Check sheet for the modelled part. Datum: model origin and axes. Units: mm. A direction names the side the tool comes from. Coordinates: 2 decimals unless noted, no trailing zeros. Order: outer loops, then holes, each group sorted by start corner. A loop starts at its lowest first (then second) coordinate and runs counter-clockwise, first axis right, second up. Notation, with made-up numbers: (83, 16.5) -> (114, 16.5) arc R25 cw to (114, 42.5) -> close; hole circle Ø6 at (87, 44). An arc over 180 degrees is marked (long way). Put each result on its own line as item: value. Start each with the question number.
```python
from build123d import *

# Parameters (mm, degrees)
F0_W     = 254
F0_H     = 254
F0_R     = 12.7
F1_DEPTH = 38.1
F2_W     = 254
F2_H     = 254
F2_W_2   = 241.3
F2_H_2   = 241.3
F3_DEPTH = 25.4
F4_R     = 19.05
F5_DEPTH = 37.846
F7_DEPTH = 50.8
F9_DEPTH = 50.8


with BuildPart() as f1:
    # F0 (on Top) → F1 (new body)
    with BuildSketch(Plane.XY):
        Rectangle(F0_W, F0_H)
        Circle(F0_R, mode=Mode.SUBTRACT)
    extrude(amount=-F1_DEPTH)

    # F2 (on face) → F3 (join)
    with BuildSketch(Plane.XY):
        Rectangle(F2_W, F2_H)
        Rectangle(F2_W_2, F2_H_2, mode=Mode.SUBTRACT)
    extrude(amount=F3_DEPTH)

    # F4 (on face) → F5 (cut)
    with BuildSketch(Plane.XY):
        Circle(F4_R)
    extrude(amount=-F5_DEPTH, mode=Mode.SUBTRACT)

    # F6 (on face) → F7 (join)
    with BuildSketch(Plane.YZ.offset(127)):
        Polygon((203.2, -170.082272), (127, -38.1), (76.2, -38.1), (152.4, -170.082272), align=None)
        Polygon((-76.2, -38.1), (-127, -38.1), (-203.2, -170.082272), (-152.4, -170.082272), align=None)
    extrude(amount=-F7_DEPTH)

    # F8 (on face) → F9 (join)
    with BuildSketch(Plane(origin=(-127, 0, 0), x_dir=(0, -1, 0), z_dir=(-1, 0, 0))):
        Polygon((-76.2, -38.1), (-127, -38.1), (-203.2, -170.082272), (-152.4, -170.082272), align=None)
        Polygon((203.2, -170.082272), (127, -38.1), (76.2, -38.1), (152.4, -170.082272), align=None)
    extrude(amount=-F9_DEPTH)


solid = f1.part
```
1) Access from +Z, -Z, +X, -X, +Y, -Y to the whole of each face (thin tool, end or side, straight path). Record for faces 1 (the flat face through (26, 2, -38.1)), 2 (the flat face through (76.2, -141, -103)), 3 (the flat face through (-29, 2, 0)), 4 (the flat face through (-101.956, 114.833, -105.015)), 5 (the flat face through (-2, -127, -7)).
2) Sectioned sample at D-D (x = -72). Record the boundary of the cut face in (y, z), plus the area to 4 significant figures.
3) Mould release check, pull along X, two halves, no side actions. Record for faces 6 (the flat face through (101.96, 113.77, -103.17)), 7 (the flat face through (-127, 1, -21)), 8 (the flat face through (-76.2, 141, -103)): +X half, -X half, draft (parallel to the pull), parting line (faces both ways), or undercut.
4) Scan lines: line 1 along Y through (x, z) = (0, -15.5); line 2 along X through (y, z) = (-172, -146); line 3 along Z through (x, y) = (-84, -46.5). Record each from-to range of solid material in increasing order. Write a range as [from, to].
5) Sectioned sample at A-A (y = 0). Record the boundary of the cut face in (x, z), plus the area to 3 significant figures.
6) Sectioned sample at C-C (z = 6.5). Record the boundary of the cut face in (x, y), plus the area to 3 significant figures.
7) Gauge pin test, flat ends, axial feed: pin 1 (8 mm diameter, centred on x = -6, y = 42.5, fed in from +Z); pin 2 (5 mm diameter, centred on x = 77.5, y = -109.5, fed in from -Z); pin 3 (12.5 mm diameter, centred on x = 44.5, z = 10, fed in from -Y). Record the tip position at first contact, or that the pin passes through.
Entries:
1. face 1: -Z
1. face 2: -Z, +Y, -Y
1. face 3: +Z
1. face 4: -Z, +X, -X
1. face 5: +Z, +X, -X, -Y
2. outline: (-127, -38.1) -> (127, -38.1) -> (127, 25.4) -> (120.65, 25.4) -> (120.65, 0) -> (-120.65, 0) -> (-120.65, 25.4) -> (-127, 25.4) -> close
2. area: 10,000 mm2
3. face 6: draft
3. face 7: -X half
3. face 8: undercut
4. line 1: y = [-127, -19.05], [19.05, 127]
4. line 2: x = [-127, -76.2], [76.2, 127]
4. line 3: z = [-38.1, 0]
5. outline: (-127, -38.1) -> (-12.7, -38.1) -> (-12.7, -37.85) -> (-19.05, -37.85) -> (-19.05, 0) -> (-120.65, 0) -> (-120.65, 25.4) -> (-127, 25.4) -> close; (12.7, -38.1) -> (127, -38.1) -> (127, 25.4) -> (120.65, 25.4) -> (120.65, 0) -> (19.05, 0) -> (19.05, -37.85) -> (12.7, -37.85) -> close
5. area: 8,550 mm2
6. outline: (-127, -127) -> (127, -127) -> (127, 127) -> (-127, 127) -> close; hole (-120.65, -120.65) -> (120.65, -120.65) -> (120.65, 120.65) -> (-120.65, 120.65) -> close
6. area: 6,290 mm2
7. pin 1: stops at z = 0
7. pin 2: stops at z = -100.11
7. pin 3: stops at y = -127
